Design review of the part built by this model. Coordinates are the model's own, in mm. A direction names the side the tool comes from. Give positions to 0.01 mm unless a question says otherwise; leave off trailing zeros. Loops run counter-clockwise (first coordinate to the right, second up) from the corner with the lowest first, then second, coordinate; pieces in that order, holes last.
from build123d import *

# Parameters (mm, degrees)
CUT_EXTRUDE_START                    = 15
SKETCH_4_W                           = 227.596726831
SKETCH_4_H                           = 99.432892292
CUT_EXTRUDE_1_DEPTH                  = 50
CUT_EXTRUDE_2_REACH                  = 160.114
SKETCH_5_R                           = 20
CUT_EXTRUDE_4_REACH                  = 157.965
CUT_EXTRUDE_4_END_RADIUS             = 10
SKETCH_6_W                           = 20
SKETCH_6_H                           = 5
CUT_EXTRUDE_4_DIRECTION_2_REACH      = 157.965
CUT_EXTRUDE_4_DIRECTION_2_END_RADIUS = 10
CUT_EXTRUDE_5_REACH                  = 159.321
SKETCH_8_R                           = 5
RIB_1_REACH                          = 157.965
SKETCH_9_WALL_W                      = 352.18110561
SKETCH_9_WALL_H                      = 10


with BuildPart() as part:
    # 草图2 → 旋转1 (revolve)
    with BuildSketch(Plane.XY, mode=Mode.PRIVATE) as revolve_1_sk:
        with BuildLine():
            Line((35.968736425, 17.5), (102.009618943, 17.5))
            Line((102.009618943, 17.5), (115, 10))
            Line((115, 10), (150, 10))
            Line((150, 10), (150, 0))
            Line((150, 0), (40, 0))
            Line((40, 0), (-40, 0))
            ThreePointArc((-40, 0), (-8.979157617, 38.979157617), (35.968736425, 17.5))
        make_face()
    revolve(revolve_1_sk.sketch.rotate(Axis((0, 0, 0), (1, 0, 0)), 90), axis=Axis((0, 0, 0), (1, 0, 0)))

    # 草图4 → 切除-拉伸1 (cut)
    with BuildSketch(Plane.XY.offset(CUT_EXTRUDE_START)):
        with Locations((54.933799673, 2.64801311)):
            Rectangle(SKETCH_4_W, SKETCH_4_H)
    cut_extrude_1 = extrude(amount=CUT_EXTRUDE_1_DEPTH, mode=Mode.SUBTRACT)

    # 镜向1: 切除-拉伸1 across plane
    add(cut_extrude_1.mirror(Plane.XY), mode=Mode.SUBTRACT)

    # 草图5 → 切除-拉伸2 (cut, up to next)
    with BuildSketch(Plane.XY.offset(15), mode=Mode.PRIVATE) as cut_extrude_2_sk1:
        Circle(SKETCH_5_R)
    cut_extrude_2_tool1 = extrude(cut_extrude_2_sk1.sketch, amount=-CUT_EXTRUDE_2_REACH, mode=Mode.PRIVATE) & part.part
    add(cut_extrude_2_tool1.solids().sort_by_distance((0, 0, 15))[0], mode=Mode.SUBTRACT)

    # 切除-拉伸4: up to this cylinder (the profile starts inside it)
    cut_extrude_4_end = Plane(origin=(140, 0, 0), z_dir=(-1, 0, 0)) * Cylinder(CUT_EXTRUDE_4_END_RADIUS, 336.93, mode=Mode.PRIVATE)
    # 草图6 → 切除-拉伸4 (cut, up to the surface)
    with BuildSketch(Plane.XY, mode=Mode.PRIVATE) as cut_extrude_4_sk1:
        with Locations((140, 7.5)):
            Rectangle(SKETCH_6_W, SKETCH_6_H)
    cut_extrude_4_tool1 = extrude(cut_extrude_4_sk1.sketch, amount=-CUT_EXTRUDE_4_REACH, mode=Mode.PRIVATE) & cut_extrude_4_end
    add(cut_extrude_4_tool1.solids().sort_by_distance((140, 7.5, 0))[0], mode=Mode.SUBTRACT)
    # 草图6 → 切除-拉伸4 (cut, up to the surface)
    with BuildSketch(Plane.XY, mode=Mode.PRIVATE) as cut_extrude_4_sk2:
        with Locations((140, -7.5)):
            Rectangle(SKETCH_6_W, SKETCH_6_H)
    cut_extrude_4_tool2 = extrude(cut_extrude_4_sk2.sketch, amount=-CUT_EXTRUDE_4_REACH, mode=Mode.PRIVATE) & cut_extrude_4_end
    add(cut_extrude_4_tool2.solids().sort_by_distance((140, -7.5, 0))[0], mode=Mode.SUBTRACT)

    # 切除-拉伸4 direction 2: up to this cylinder (the profile starts inside it)
    cut_extrude_4_direction_2_end = Plane(origin=(140, 0, 0), z_dir=(-1, 0, 0)) * Cylinder(CUT_EXTRUDE_4_DIRECTION_2_END_RADIUS, 336.93, mode=Mode.PRIVATE)
    # 草图6 → 切除-拉伸4 direction 2 (cut, up to the surface)
    with BuildSketch(Plane.XY, mode=Mode.PRIVATE) as cut_extrude_4_direction_2_sk1:
        with Locations((140, 7.5)):
            Rectangle(SKETCH_6_W, SKETCH_6_H)
    cut_extrude_4_direction_2_tool1 = extrude(cut_extrude_4_direction_2_sk1.sketch, amount=CUT_EXTRUDE_4_DIRECTION_2_REACH, mode=Mode.PRIVATE) & cut_extrude_4_direction_2_end
    add(cut_extrude_4_direction_2_tool1.solids().sort_by_distance((140, 7.5, 0))[0], mode=Mode.SUBTRACT)
    # 草图6 → 切除-拉伸4 direction 2 (cut, up to the surface)
    with BuildSketch(Plane.XY, mode=Mode.PRIVATE) as cut_extrude_4_direction_2_sk2:
        with Locations((140, -7.5)):
            Rectangle(SKETCH_6_W, SKETCH_6_H)
    cut_extrude_4_direction_2_tool2 = extrude(cut_extrude_4_direction_2_sk2.sketch, amount=CUT_EXTRUDE_4_DIRECTION_2_REACH, mode=Mode.PRIVATE) & cut_extrude_4_direction_2_end
    add(cut_extrude_4_direction_2_tool2.solids().sort_by_distance((140, -7.5, 0))[0], mode=Mode.SUBTRACT)

    # 草图8 → 切除-拉伸5 (cut, up to next)
    with BuildSketch(Plane(origin=(0, 5, 0), x_dir=(1, 0, 0), z_dir=(0, 1, 0)), mode=Mode.PRIVATE) as cut_extrude_5_sk1:
        with Locations(Location((140, 0, 0), (0, 0, 270))):
            Circle(SKETCH_8_R)
    cut_extrude_5_tool1 = extrude(cut_extrude_5_sk1.sketch, amount=-CUT_EXTRUDE_5_REACH, mode=Mode.PRIVATE) & part.part
    add(cut_extrude_5_tool1.solids().sort_by_distance((140, 5, 0))[0], mode=Mode.SUBTRACT)

    # 草图9 wall → 筋1 (add, up to next)
    with BuildSketch(Plane(origin=(47.508055761, 22.5, 0), x_dir=(0.965223306875, -0.261426792555, 0), z_dir=(0.261426792555, 0.965223306875, 0)), mode=Mode.PRIVATE) as rib_1_sk1:
        Rectangle(SKETCH_9_WALL_W, SKETCH_9_WALL_H)
    rib_1_tool1 = extrude(rib_1_sk1.sketch, amount=-RIB_1_REACH, mode=Mode.PRIVATE) - part.part
    rib_1 = rib_1_tool1.solids().sort_by_distance((47.508055761, 22.5, 0))[0]
    add(rib_1)

    # 镜向2: 筋1 across plane
    add(rib_1.mirror(Plane(origin=(0, 0, 0), x_dir=(0, 0, 1), z_dir=(0, -1, 0))))


solid = part.part
Q1. Draft analysis for pull direction X (two halves, no side actions). For faces 1 (the face through (69.45, 17.5, -0.25)), 2 (the face through (114.369, 9.195, 4.782)), 3 (the face through (-4.336, -19.524, 0.21)), state which applies: pulls with the +X half, pulls with the -X half, needs draft (parallel to the pull), parting line crosses it, or undercut.
Results:
face 1: needs draft
face 2: pulls with the +X half
face 3: undercut
Q2. Take a section at C-C (z = 0). Give the boundary of the cut face in (x, y), plus the area to 3 significant figures.
Results:
outline: (29.05, -27.5) - (65.97, -17.5) - (102.01, -17.5) - (115, -10) - (130, -10) - (130, -5) - (135, -5) - (135, 5) - (130, 5) - (130, 10) - (115, 10) - (102.01, 17.5) - (65.97, 17.5) - (29.05, 27.5) arc R40 ccw (long way) to start; (145, -5) - (150, -5) - (150, 5) - (145, 5) - close; hole circle Ø40 at (0, 0)
area: 7,040 mm2
Q3. Tool access review of faces 4 (the face through (43, -21, 5)), 5 (the face through (130, -7, 0)), 6 (the face through (69.45, -17.5, 0.25)), 7 (the face through (43, 21, -5)), 8 (the face through (43, -21, -5)): name each direction out of +Z, -Z, +X, -X, +Y, -Y from which nothing blocks a thin tool from reaching the whole face with its end or side.
Results:
face 4: +Z, +X, -Y
face 5: +Z, -Z, +X, -Y
face 6: +X, -Y
face 7: -Z, +X, +Y
face 8: -Z, +X, -Y
Q4. Take a section at B-B (x = 140). Give the boundary of the cut face in (y, z).
Results:
outline: (-5, -8.66) arc R10 ccw to (5, -8.66) - (5, -5) - (-5, -5) - close; (-5, 5) - (5, 5) - (5, 8.66) arc R10 ccw to (-5, 8.66) - close
Q5. Wall thickness on line 1 (X direction, y = -1, z = 0); line 2 (X direction, y = -1.5, z = 0); line 3 (Z direction, x = 75.5, y = -15): over which ranges is each line inside the solid? List them lowest first.
Results:
line 1: x = -39.99 to -19.97, 19.97 to 135, 145 to 150
line 2: x = -39.97 to -19.94, 19.94 to 135, 145 to 150
line 3: z = -9.01 to 9.01
Q6. Take a section at A-A (y = 0). Give the boundary of the cut face in (x, z), plus the area to 3 significant figures.
Results:
outline: (-37.08, -15) - (-20, -15) - (-20, 15) - (-37.08, 15) arc R40 ccw to start; (20, -15) - (106.34, -15) - (115, -10) - (150, -10) - (150, 10) - (115, 10) - (106.34, 15) - (20, 15) - close; hole circle Ø10 at (140, 0)
area: 4,000 mm2
Q7. Insertion check: pin 1 (5 mm diameter, centred on x = 82, z = -9.5, fed in from -Y); pin 2 (13 mm diameter, centred on x = 140, z = 0, fed in from -Y); pin 3 (1 mm diameter, centred on y = 30, z = -7, fed in from -X). Each pin has a flat end and moves straight along its axis. Give the tip position at first contact, or say it passes through.
Results:
pin 1: stops at y = -16.04
pin 2: stops at y = -5
pin 3: stops at x = -26.11
Q8. Take a section at D-D (x = 0). Give the boundary of the cut face in (y, z).
Results:
outline: (-37.08, -15) - (-20, -15) - (-20, 15) - (-37.08, 15) arc R40 ccw to start; (20, -15) - (37.08, -15) arc R40 ccw to (37.08, 15) - (20, 15) - close
